Part model, mm, in its own coordinate system. Face numbers are marked on the shaded views. A direction names the side the tool comes from. Round coordinates to 2 decimals unless told otherwise and drop trailing zeros. Order: outer loops, then holes, each group sorted by start corner. A loop starts at its lowest first (then second) coordinate and runs counter-clockwise, first axis right, second up. Notation, with made-up numbers: (22, 79) - (80, 79) arc R14 cw to (80, 84) - close; hole circle Ø6 at (54.25, -16). An arc over 180 degrees is marked (long way). Return JSON: item names as keys, results as strings. Group by question number.
Item 1: Probe probe 1 along Z at (x, y) = (0, -15.2); probe 2 along Z at (x, y) = (20.5, -4.5); probe 3 along Y at (x, z) = (14.5, 12). List the from-to ranges inside material, lowest first.
Item 2: Saw through at A-A on x = 0. List the corners of the cut face in (y, z).
Item 3: Tool access for the marked faces 4 and 5: list every direction of +Z, -Z, +X, -X, +Y, -Y with a clear straight run to the whole face (end or side of a thin tool).
Item 4: Two-plate mould, pull along Z, no slides. Class the marked faces 1, 2 and 3: released by +Z, released by -Z, zero draft, split by the parting line, or undercut.
Item 5: Saw through at D-D on x = 10. List the corners of the cut face in (y, z).
Item 6: Drop flat-ended pins along their axis: pin 1 (3 mm diameter, centred on x = 0, z = 0, fed in from +Y); pin 2 (5 mm diameter, centred on x = 18.5, z = -12, fed in from +Y); pin 3 (7.5 mm diameter, centred on y = -8.5, z = 6, fed in from +X). Give the stop position or say it passes through.
Item 7: Saw through at B-B on z = 0. List the corners of the cut face in (x, y), and give its area (3 significant figures).
Item 8: Saw through at C-C on y = -10.5. List the corners of the cut face in (x, z), and give its area (3 significant figures).
```python
from build123d import *

# Parameters (mm, degrees)
F0_W     = 48.26
F0_H     = 38.1
F1_DEPTH = 15.24
F3_T     = -0.254
F4_D     = 6.858
F6_D     = 5.08
F7_W     = 8.128
F7_H     = 3.048
F8_DEPTH = 25.4


with BuildPart() as f1:
    # F0 (on Front) → F1 (new body)
    with BuildSketch(Plane.XZ):
        Rectangle(F0_W, F0_H)
    extrude(amount=F1_DEPTH)

    # F3
    f3_openings = [f1.faces().sort_by_distance(p)[0] for p in [
        (0, 0, 0),
        (24.13, -7.62, 0),
    ]]
    offset(amount=F3_T, openings=f3_openings)

    # F4 (through all)
    with Locations(Plane.XZ.offset(15.24)):
        with Locations((-16.383, 0)):
            Hole(F4_D / 2)

    # F6 (through all)
    with Locations(Plane.XZ.offset(15.24)):
        with Locations((0, 0)):
            Hole(F6_D / 2)

    # F7 (on face) → F8 (cut)
    with BuildSketch(Plane.XY.offset(19.05)):
        with Locations((16.256, -11.051697)):
            Rectangle(F7_W, F7_H)
    extrude(amount=-F8_DEPTH, mode=Mode.SUBTRACT)


solid = f1.part
```
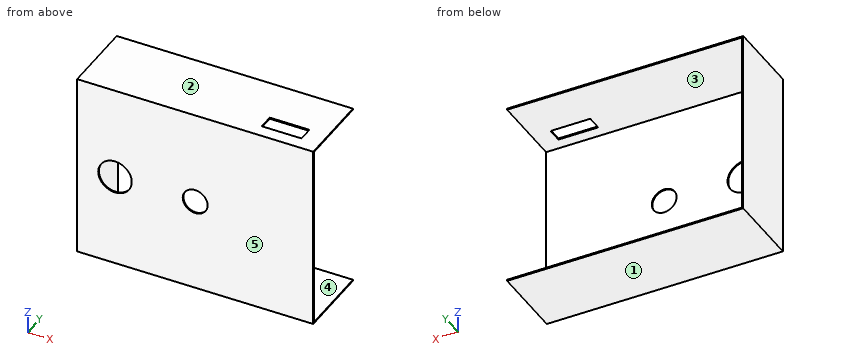
Filled in:
{
 "1": {"probe 1": "z = -19.05 to -2.54, 2.54 to 19.05", "probe 2": "z = -19.05 to -18.8, 18.8 to 19.05", "probe 3": "y = -15.24 to -14.99"},
 "2": {"outline": "(-15.24, -19.05) - (0, -19.05) - (0, -18.8) - (-14.99, -18.8) - (-14.99, -2.54) - (-15.24, -2.54) - close; (-15.24, 2.54) - (-14.99, 2.54) - (-14.99, 18.8) - (0, 18.8) - (0, 19.05) - (-15.24, 19.05) - close"},
 "3": {"face 4": "+X, +Y", "face 5": "+Z, -Z, +X, -X, -Y"},
 "4": {"face 1": "released by -Z", "face 2": "released by +Z", "face 3": "undercut"},
 "5": {"outline": "(-15.24, -19.05) - (0, -19.05) - (0, -18.8) - (-14.99, -18.8) - (-14.99, 18.8) - (0, 18.8) - (0, 19.05) - (-15.24, 19.05) - close"},
 "6": {"pin 1": "passes through", "pin 2": "stops at y = -14.99", "pin 3": "stops at x = -23.88"},
 "7": {"outline": "(-24.13, -15.24) - (-19.81, -15.24) - (-19.81, -14.99) - (-23.88, -14.99) - (-23.88, 0) - (-24.13, 0) - close; (-12.95, -15.24) - (-2.54, -15.24) - (-2.54, -14.99) - (-12.95, -14.99) - close; (2.54, -15.24) - (24.13, -15.24) - (24.13, -14.99) - (2.54, -14.99) - close", "area": "13.0 mm^2"},
 "8": {"outline": "(-24.13, -19.05) - (24.13, -19.05) - (24.13, -18.8) - (-23.88, -18.8) - (-23.88, 18.8) - (12.19, 18.8) - (12.19, 19.05) - (-24.13, 19.05) - close; (20.32, 18.8) - (24.13, 18.8) - (24.13, 19.05) - (20.32, 19.05) - close", "area": "32.0 mm^2"}
}
